from build123d import *

# Parameters (mm, degrees)
SKETCH1_R           = 15
SKETCH1_R_2         = 6
BOSS_EXTRUDE1_DEPTH = 30


with BuildPart() as part:
    # Sketch1 → Boss-Extrude1 (new body)
    with BuildSketch(Plane.XY):
        with BuildLine():
            Line((-59.555920585, -15.55654054), (95.444079415, -15.55654054))
            Line((95.444079415, -15.55654054), (95.444079415, 6.44345946))
            ThreePointArc((95.444079415, 6.44345946), (93.100933664, 12.100313709), (87.444079415, 14.44345946))
            Line((87.444079415, 14.44345946), (57.445626465, 14.44345946))
            ThreePointArc((57.445626465, 14.44345946), (52.193369151, 16.409075224), (49.522091781, 21.340011184))
            ThreePointArc((49.522091781, 21.340011184), (35.491805322, 49.661803472), (7.279378806, 63.910727872))
            ThreePointArc((7.279378806, 63.910727872), (2.389428109, 66.596609718), (0.444079415, 71.825490818))
            Line((0.444079415, 71.825490818), (0.444079415, 86.44345946))
            ThreePointArc((0.444079415, 86.44345946), (-1.899066336, 92.100313709), (-7.555920585, 94.44345946))
            Line((-7.555920585, 94.44345946), (-51.555920585, 94.44345946))
            ThreePointArc((-51.555920585, 94.44345946), (-57.212774835, 92.100313709), (-59.555920585, 86.44345946))
            Line((-59.555920585, 86.44345946), (-59.555920585, -15.55654054))
        make_face()
        with Locations((-29.555920585, 74.44345946)):
            Circle(SKETCH1_R, mode=Mode.SUBTRACT)
        with Locations((-40, -0.55654054)):
            Circle(SKETCH1_R_2, mode=Mode.SUBTRACT)
        with Locations((-20, -0.55654054)):
            Circle(SKETCH1_R_2, mode=Mode.SUBTRACT)
        with Locations((0, -0.55654054)):
            Circle(SKETCH1_R_2, mode=Mode.SUBTRACT)
        with Locations((20, -0.55654054)):
            Circle(SKETCH1_R_2, mode=Mode.SUBTRACT)
        with Locations((40, -0.55654054)):
            Circle(SKETCH1_R_2, mode=Mode.SUBTRACT)
        with Locations((60, -0.55654054)):
            Circle(SKETCH1_R_2, mode=Mode.SUBTRACT)
        with Locations((80, -0.55654054)):
            Circle(SKETCH1_R_2, mode=Mode.SUBTRACT)
        with BuildLine():
            Line((0, 44.44345946), (-32, 44.44345946))
            ThreePointArc((-32, 44.44345946), (-37.656854249, 42.100313709), (-40, 36.44345946))
            Line((-40, 36.44345946), (-40, 22.44345946))
            ThreePointArc((-40, 22.44345946), (-37.656854249, 16.78660521), (-32, 14.44345946))
            Line((-32, 14.44345946), (20.493901532, 14.44345946))
            ThreePointArc((20.493901532, 14.44345946), (27.099684123, 17.930850861), (27.946229362, 25.352550369))
            ThreePointArc((27.946229362, 25.352550369), (16.922282245, 39.215144175), (0, 44.44345946))
        make_face(mode=Mode.SUBTRACT)
    extrude(amount=BOSS_EXTRUDE1_DEPTH)


solid = part.part
Input: part model. Units: mm. Frame: model coordinates. A direction names the side the tool comes from. Give positions to 0.01 mm unless a question says otherwise; leave off trailing zeros. Write each loop counter-clockwise with the first axis right and the second up, starting at its lowest first coordinate (ties: lowest second). Pieces come first, ordered by that corner, then holes.
Q1. Set-up query: faces 5 (the face through (73, 14.443, 15)), 6 (the face through (95.444, -5, 15)), 7 (the face through (-37.594, 42.162, 14.79)). Return all of +Z, -Z, +X, -X, +Y, -Y with unobstructed straight access to the full face (end or side cutting, diameter ignored); none if empty.
Q2. Section B-B, the plane y = 18. Output: boundary loops of the cut face in (x, z), plus the area to 3 significant figures.
Q3. First-contact query: P1, Ø8, axis at y = 41, z = 22, coming from the +X side; P2, Ø11, axis at y = 26, z = 14, coming from the +X side; P3, Ø4.5, axis at y = 79.5, z = 16, coming from the +X side; P4, Ø1, axis at x = -20.5, y = 3.5, coming from the +Z side. Flat tips, straight axial feed; report the tip coordinate or a pass-through.
Q4. Section D-D, the plane y = 1. State how many separate pieces and enclosed holes the cut face has, plus the area to 3 significant figures.
Q5. Section A-A, the plane x = 60. Output: boundary loops of the cut face in (y, z), plus the area to 3 significant figures.
Q6. Material intervals for probe 1 along Y at (x, z) = (-20, 18.75); probe 2 along X at (y, z) = (75.5, 28); probe 3 along Y at (x, z) = (-41, 18.25), sorted ascending.
Q7. Section C-C, the plane x = 23. Output: boundary loops of the cut face in (y, z).
Q8. Pull-direction query (X, two-part tool) for faces 1 (the face through (-29, 94.443, 15)), 2 (the face through (-40, 30, 15)), 3 (the face through (54.006, -0.293, 14.79)), 4 (the face through (93.2, 12, 14.8)); classes: pulls with the +X half, pulls with the -X half, needs draft (parallel to the pull), parting line crosses it, or undercut.
Filled in:
1. face 5: +Z, -Z, +X, +Y
1. face 6: +Z, -Z, +X, +Y, -Y
1. face 7: +Z, -Z
2. outline: (-59.56, 0) - (-38.65, 0) - (-38.65, 30) - (-59.56, 30) - close; (27.15, 0) - (50.79, 0) - (50.79, 30) - (27.15, 30) - close
2. area: 1,340 mm2
3. P1: stops at x = 44.62
3. P2: stops at x = 49.69
3. P3: stops at x = 0.44
3. P4: passes through
4. separate pieces: 8
4. enclosed holes: 0
4. area: 2,220 mm2
5. outline: (-15.56, 0) - (-6.56, 0) - (-6.56, 30) - (-15.56, 30) - close; (5.44, 0) - (14.44, 0) - (14.44, 30) - (5.44, 30) - close
5. area: 540 mm2
6. probe 1: y = -15.56 to -6.56, 5.44 to 14.44, 44.44 to 62.88, 86.01 to 94.44
6. probe 2: x = -59.56 to -44.52, -14.59 to 0.44
6. probe 3: y = -15.56 to -6.47, 5.36 to 64.75, 84.14 to 94.44
7. outline: (-15.56, 0) - (-5.75, 0) - (-5.75, 30) - (-15.56, 30) - close; (4.64, 0) - (14.85, 0) - (14.85, 30) - (4.64, 30) - close; (33.7, 0) - (58.84, 0) - (58.84, 30) - (33.7, 30) - close
8. face 1: needs draft
8. face 2: undercut
8. face 3: undercut
8. face 4: pulls with the +X half
